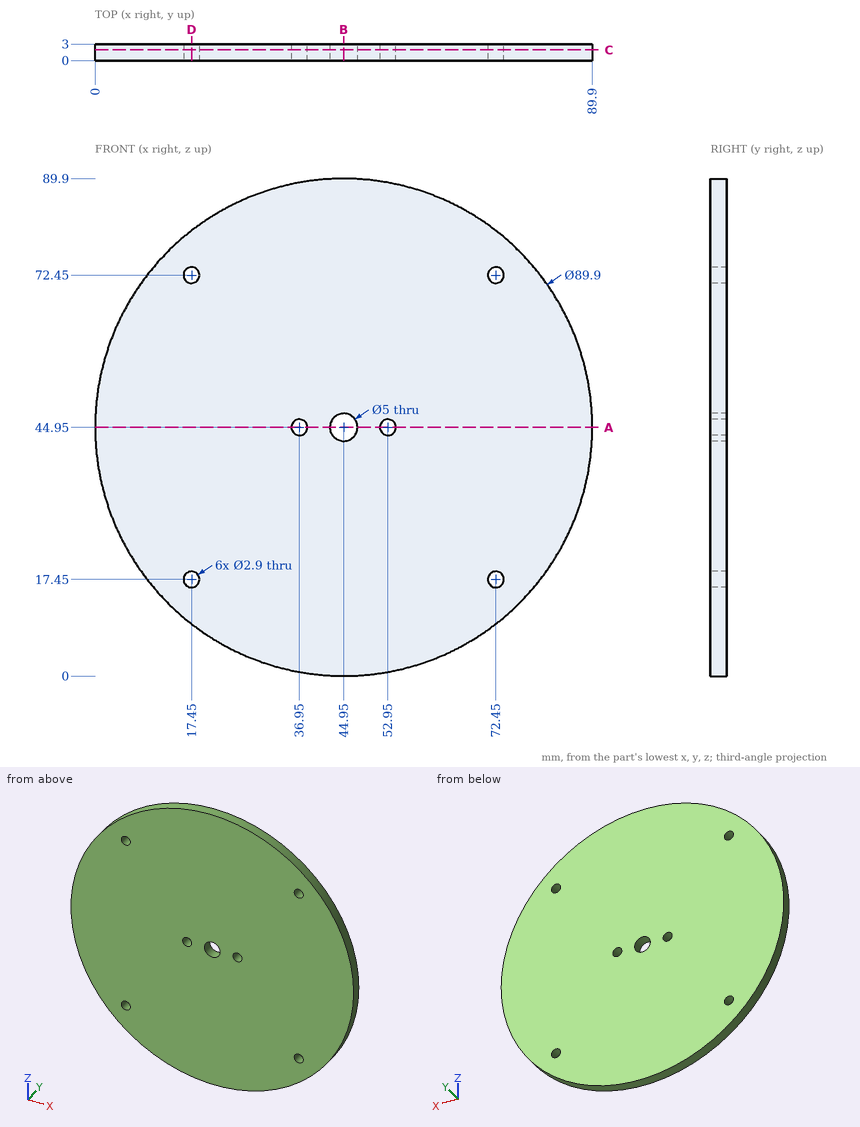
Source: three-view drawing plus pictorial views. Frame: mm from the lowest corner of the part. Coordinates: 2 decimals unless noted, no trailing zeros. Loops run counter-clockwise (first coordinate to the right, second up) from the corner with the lowest first, then second, coordinate; pieces in that order, holes last. Notation, with made-up numbers: (-24.5, 68.25) -> (2.5, 68.25) arc R31 ccw to (2.5, 104.25) -> close; hole circle Ø9 at (39, 43.25). An arc over 180 degrees is marked (long way). Answer in a Markdown table with one row per item. Add a question column.
Q1. Section C-C on y = 1.95. Return the cut outline in (x, z), and give its area (3 significant figures).
Q2. Contact query for flat-ended pins moving along their axis: pin 1 Ø1.5 at (y, z) = (1.5, 50) entering from +X; pin 2 Ø1.7 at (x, z) = (52.95, 44.95) entering from +Y. Output: stop coordinate, or through.
Q3. Ray query, line 1 along Z through (x, y) = (72.45, 2.45); line 2 along Z through (x, y) = (44.95, 0.95). Return the intervals inside material, ascending.
Q4. Section B-B on x = 44.95. Return the cut outline in (y, z), and give its area (3 significant figures).
Q5. Section D-D on x = 17.45. Return the cut outline in (y, z).
Q6. Section A-A on z = 44.95. Return the cut outline in (x, y), and give its area (3 significant figures).
Computed values:
| question | item | result |
|---|---|---|
| 1 | outline | circle Ø89.9 at (44.95, 44.95); hole circle Ø2.9 at (17.45, 17.45); hole circle Ø2.9 at (17.45, 72.45); hole circle Ø2.9 at (36.95, 44.95); hole circle Ø5 at (44.95, 44.95); hole circle Ø2.9 at (52.95, 44.95); hole circle Ø2.9 at (72.45, 17.45); hole circle Ø2.9 at (72.45, 72.45) |
| 1 | area | 6,290 mm^2 |
| 2 | pin 1 | stops at x = 89.69 |
| 2 | pin 2 | passes through |
| 3 | line 1 | z = 9.39 to 16, 18.9 to 71, 73.9 to 80.51 |
| 3 | line 2 | z = 0 to 42.45, 47.45 to 89.9 |
| 4 | outline | (0, 0) -> (3, 0) -> (3, 42.45) -> (0, 42.45) -> close; (0, 47.45) -> (3, 47.45) -> (3, 89.9) -> (0, 89.9) -> close |
| 4 | area | 255 mm^2 |
| 5 | outline | (0, 9.39) -> (3, 9.39) -> (3, 16) -> (0, 16) -> close; (0, 18.9) -> (3, 18.9) -> (3, 71) -> (0, 71) -> close; (0, 73.9) -> (3, 73.9) -> (3, 80.51) -> (0, 80.51) -> close |
| 6 | outline | (0, 0) -> (35.5, 0) -> (35.5, 3) -> (0, 3) -> close; (38.4, 0) -> (42.45, 0) -> (42.45, 3) -> (38.4, 3) -> close; (47.45, 0) -> (51.5, 0) -> (51.5, 3) -> (47.45, 3) -> close; (54.4, 0) -> (89.9, 0) -> (89.9, 3) -> (54.4, 3) -> close |
| 6 | area | 237 mm^2 |
